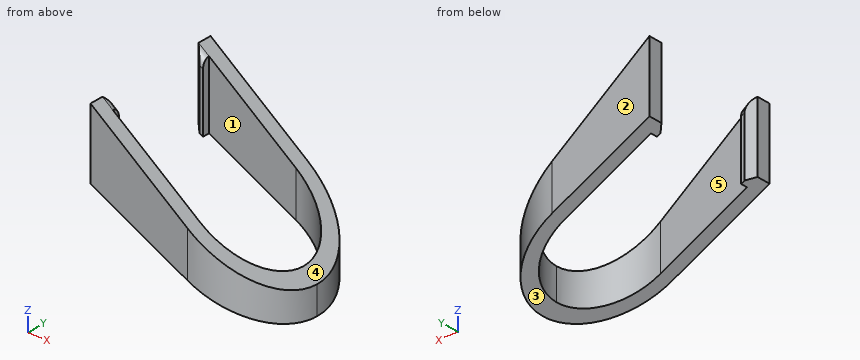
from build123d import *

# Parameters (mm, degrees)
F1_DEPTH    = 34.925
F3_DEPTH    = 31.75
F4_T1_DEPTH = 8.9296875
F4_T3_DEPTH = 8.9296875


# Not quite as in the source:
# - a fillet or chamfer that OpenCascade refuses, or shapes differently, is made with other operations: its cross-section is extruded or revolved along the edge and cut away or added


with BuildPart() as f1:
    # F0 (on Top) → F1 (new body)
    with BuildSketch(Plane.XY):
        with BuildLine():
            Line((0, 15.875), (-22.225, 15.875))
            Line((-22.225, 15.875), (-22.225, 12.7))
            Line((-22.225, 12.7), (-20.6375, 11.1125))
            Line((-20.6375, 11.1125), (-19.84375, 11.1125))
            Line((-19.84375, 11.1125), (-19.84375, 12.7))
            Line((-19.84375, 12.7), (0, 12.7))
            ThreePointArc((0, 12.7), (8.9802561211, 8.9802561211), (12.7, 0))
            ThreePointArc((12.7, 0), (8.9802561211, -8.9802561211), (0, -12.7))
            Line((0, -12.7), (-19.84375, -12.7))
            Line((-19.84375, -12.7), (-19.84375, -11.1125))
            Line((-19.84375, -11.1125), (-20.6375, -11.1125))
            Line((-20.6375, -11.1125), (-22.225, -12.7))
            Line((-22.225, -12.7), (-22.225, -15.875))
            Line((-22.225, -15.875), (0, -15.875))
            ThreePointArc((0, -15.875), (11.2253201513, -11.2253201513), (15.875, 0))
            ThreePointArc((15.875, 0), (11.2253201513, 11.2253201513), (0, 15.875))
        make_face()
    extrude(amount=F1_DEPTH)

    # F2 (on face) → F3 (cut, through all)
    with BuildSketch(Plane.XZ.offset(15.875)):
        Polygon((0, 18.25625), (0, 34.925), (-22.225, 34.925), align=None)
        Polygon((15.875, 6.35), (15.875, 34.925), (0, 34.925), (0, 18.25625), align=None)
        Polygon((-22.225, 0), (0, 0), (0, 7.9375), (-22.225, 19.05), align=None)
        Polygon((0, 0), (15.875, 0), (0, 7.9375), align=None)
    extrude(amount=-F3_DEPTH, mode=Mode.SUBTRACT)

    # F4: fillet of radius 1.5875 on 2 edges, made by hand

    # F4_s2 → F4_t1 (cut)
    with BuildSketch(Plane(origin=(-25.43175, 0, 19.0738125), x_dir=(0, 1, 0), z_dir=(-0.8, 0, 0.6))):
        with BuildLine():
            ThreePointArc((12.7, -14.605), (11.5774679849, -14.1400320151), (11.1125, -13.0175))
            Line((11.1125, -13.0175), (11.1125, -14.605))
            Line((11.1125, -14.605), (12.7, -14.605))
        make_face()
    extrude(amount=F4_T1_DEPTH, mode=Mode.SUBTRACT)

    # F4_s4 → F4_t3 (cut)
    with BuildSketch(Plane(origin=(-32.5755, 0, 24.431625), x_dir=(0, 1, 0), z_dir=(0.8, 0, -0.6))):
        with BuildLine():
            ThreePointArc((-12.7, 14.605), (-11.5774679849, 14.1400320151), (-11.1125, 13.0175))
            Line((-11.1125, 13.0175), (-11.1125, 14.605))
            Line((-11.1125, 14.605), (-12.7, 14.605))
        make_face()
    extrude(amount=F4_T3_DEPTH, mode=Mode.SUBTRACT)


solid = f1.part
Model file for the job. Use its own axes, mm. Face numbers are marked on the shaded views. A direction names the side the tool comes from. Give positions to 0.01 mm unless a question says otherwise; leave off trailing zeros. Order: outer loops, then holes, each group sorted by start corner. A loop starts at its lowest first (then second) coordinate and runs counter-clockwise, first axis right, second up. Notation, with made-up numbers: M -1.5,71.25 L 27.5,71.25 A24 ccw 27.5,108.25 Z; hole C 20.25,-16.5 d7. An arc over 180 degrees is marked long. Write item = value, one per line.
Q1. Cut at A-A, the plane x = -18. List the corners of the cut face in (y, z) (1 decimal), then the cut area to 3 significant figures.
Derived:
outline = M -15.9,16.9 L -12.7,16.9 L -12.7,31.8 L -15.9,31.8 Z; M 12.7,16.9 L 15.9,16.9 L 15.9,31.8 L 12.7,31.8 Z
area = 94.1 mm2
Q2. Cut at D-D, the plane z = 3.5. List the corners of the cut face in (x, y) (3 decimals), then the cut area to 3 significant figures.
Derived:
outline = M 8.875,-13.162 A15.875 ccw 8.875,13.162 L 8.875,9.084 A12.7 cw 8.875,-9.084 Z
area = 81.6 mm2
Q3. Cut at B-B, the plane z = 14. List the corners of the cut face in (x, y) (3 decimals).
Derived:
outline = M -12.125,-15.875 L 0,-15.875 A15.875 ccw 5.675,-14.826 L 5.675,-11.362 A12.7 cw 0,-12.7 L -12.125,-12.7 Z; M -12.125,12.7 L 0,12.7 A12.7 cw 5.675,11.362 L 5.675,14.826 A15.875 ccw 0,15.875 L -12.125,15.875 Z
Q4. Two-plate mould, pull along Y, no slides. Class the marked faces 1, 2 and 3: pulls with the +Y half, pulls with the -Y half, needs draft (parallel to the pull), parting line crosses it, or undercut.
Derived:
face_1 = undercut
face_2 = pulls with the +Y half
face_3 = needs draft
Q5. Cut at C-C, the plane x = -5. List the corners of the cut face in (y, z) (1 decimal).
Derived:
outline = M -15.9,10.4 L -12.7,10.4 L -12.7,22 L -15.9,22 Z; M 12.7,10.4 L 15.9,10.4 L 15.9,22 L 12.7,22 Z
Q6. Flat gauge pins, fed straight in: pin 1 (12 mm diameter, centred on x = 3.5, y = 12.5, fed in from +Z); pin 2 (8 mm diameter, centred on x = -17.5, y = 8.5, fed in from +Z); pin 3 (0.8 mm diameter, centred on y = 12, z = 22, fed in from +X). Where does each tip first touch, or does it go through?
Derived:
pin_1 = 20.13
pin_2 = 32.74
pin_3 = -19.84
Q7. Tool access for the marked faces 4 and 5: list every direction of +Z, -Z, +X, -X, +Y, -Y with a clear straight run to the whole face (end or side of a thin tool).
Derived:
face_4 = +Z, +X, +Y, -Y
face_5 = +Z, -Z
Q8. Drill centre lines: line 1 (Y direction, x = -7, z = 22) (3 decimals); line 2 (Z direction, x = -5, y = -13.5); line 3 (Z direction, x = -9, y = 14). Where is each one in solid material? Low to high. Write a range as [from, to].
Derived:
line_1 = [-15.875, -12.7], [12.7, 15.875]
line_2 = [10.44, 22.01]
line_3 = [12.44, 25.01]
